Here's how the part is built. I have some questions about the finished solid (model axes, mm). Face numbers are marked on the shaded views. A direction names the side the tool comes from. Coordinates: 2 decimals unless noted, no trailing zeros. Use a Markdown table: item, result.
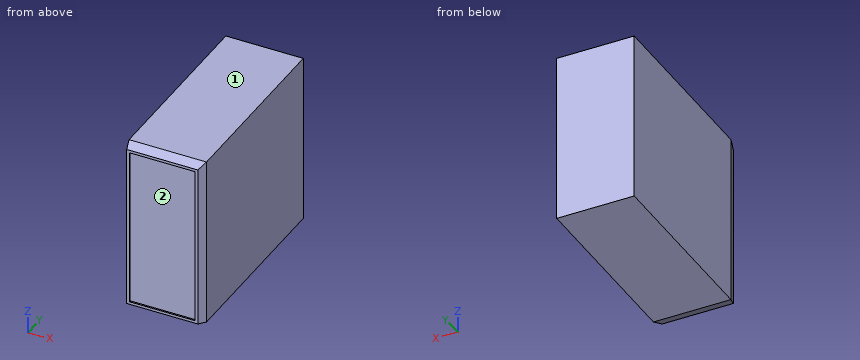
```python
from build123d import *

# Parameters (mm, degrees)
F0_W     = 184.912
F0_H     = 407.924
F1_DEPTH = 469.9
F2_SIZE2 = 25.4
F2_SIZE  = 7.62
F3_W     = 156.972
F3_H     = 379.984
F4_DEPTH = 3.81


with BuildPart() as f1:
    # F0 (on Front) → F1 (new body)
    with BuildSketch(Plane.XZ):
        with Locations((92.456, 203.962)):
            Rectangle(F0_W, F0_H)
    extrude(amount=-F1_DEPTH)

    # F2
    f2_edges = [f1.edges().sort_by_distance(p)[0] for p in [
        (0, 0, 203.962),
        (92.456, 0, 407.924),
        (184.912, 0, 203.962),
        (92.456, 0, 0),
    ]]
    f2_side = f1.faces().sort_by_distance((92.456, 0, 203.962))[0]
    chamfer(f2_edges, length=F2_SIZE, length2=F2_SIZE2, reference=f2_side)

    # F3 (on face) → F4 (cut)
    with BuildSketch(Plane.XZ):
        with Locations((92.456, 203.962)):
            Rectangle(F3_W, F3_H)
    extrude(amount=-F4_DEPTH, mode=Mode.SUBTRACT)


solid = f1.part
```
Q1. Which directions (+Z, -Z, +X, -X, +Y, -Y) give clear straight access to the entire face, cutting with the end or side of a thin tool? Please do the marked faces 1 and 2.
Check values:
| item | result |
|---|---|
| face 1 | +Z, +X, -X, +Y, -Y |
| face 2 | -Y |
Q2. Will these pins go through, and if not, where does the flat tip stop? P1, Ø3, axis at x = 99, y = 2, coming from the -Z side; P2, Ø8, axis at x = 115, z = 366.5, coming from the -Y side; P3, Ø4, axis at y = 2.5, z = 201, coming from the +X side.
Check values:
| item | result |
|---|---|
| P1 | z = 6.57 |
| P2 | y = 3.81 |
| P3 | x = 178.64 |
Q3. Please list where these lines run through material, in increasing order: L1, parallel to Y at x = 82.5, z = 94; L2, parallel to X at y = 20, z = 214. Write a range as from..to.
Check values:
| item | result |
|---|---|
| L1 | 3.81..469.9 |
| L2 | 1.62..183.29 |
